Input: part model. Units: mm. Frame: model coordinates. A direction names the side the tool comes from. Round coordinates to 2 decimals unless told otherwise and drop trailing zeros. Write each loop counter-clockwise with the first axis right and the second up, starting at its lowest first coordinate (ties: lowest second). Pieces come first, ordered by that corner, then holes. Notation, with made-up numbers: (-0.75, 16.5) - (56.25, 16.5) arc R23 cw to (56.25, 25.5) - close; hole circle Ø2 at (-19, 16.5). An arc over 180 degrees is marked (long way). Use one line per item in the form item = value.
Autodesk Fusion 360 part; units mm, degrees
sketch "Spacer" plane through (0, 0, 0) normal (0, 1, 0) x (1, 0, 0)
  line L0 (7.0148, 12.15) -> (-7.0148, 12.15)
  line L1 (-7.0148, 12.15) -> (-14.0296, 0)
  line L2 (-14.0296, 0) -> (-7.0148, -12.15)
  line L3 (-7.0148, -12.15) -> (7.0148, -12.15)
  line L4 (7.0148, -12.15) -> (14.0296, 0)
  line L5 (14.0296, 0) -> (7.0148, 12.15)
  line L6 (-12.7883, 22.15) -> (-25.5766, 0)
  line L7 (-25.5766, 0) -> (-12.7883, -22.15)
  line L8 (-12.7883, -22.15) -> (12.7883, -22.15)
  line L9 (12.7883, -22.15) -> (25.5766, 0)
  line L10 (25.5766, 0) -> (12.7883, 22.15)
  line L11 (12.7883, 22.15) -> (-12.7883, 22.15)
  line L12 (-19.1825, 11.075) -> (-10.5222, 6.075) construction
  line L13 (10.5222, 6.075) -> (19.1825, 11.075) construction
  line L14 (10.5222, -6.075) -> (19.1825, -11.075) construction
  line L15 (-10.5222, -6.075) -> (-19.1825, -11.075) construction
  circle A0 centre (-14.8523, 8.575) radius 1.45
  circle A1 centre (14.8523, 8.575) radius 1.45
  circle A2 centre (14.8523, -8.575) radius 1.45
  circle A3 centre (-14.8523, -8.575) radius 1.45
  dimension "d2" = 12.15
  dimension "d3" = 10
  dimension "d5" = 2.9
  dimension "d6" = 2.9
  dimension "d7" = 2.9
  dimension "d8" = 2.9
extrude "Extrude1" add sketch "Spacer" along normal blind 8
sketch "Lock nut hole" plane through (0, 0, 0) normal (0, 1, 0) x (1, 0, 0)
  line L0 (-11.6192, 8.575) -> (-13.2358, 11.375)
  line L1 (-13.2358, 11.375) -> (-16.4689, 11.375)
  line L2 (-16.4689, 11.375) -> (-18.0855, 8.575)
  line L3 (-18.0855, 8.575) -> (-16.4689, 5.775)
  line L4 (-16.4689, 5.775) -> (-13.2358, 5.775)
  line L5 (-13.2358, 5.775) -> (-11.6192, 8.575)
  line L6 (16.4689, 11.375) -> (13.2358, 11.375)
  line L7 (13.2358, 11.375) -> (11.6192, 8.575)
  line L8 (11.6192, 8.575) -> (13.2358, 5.775)
  line L9 (13.2358, 5.775) -> (16.4689, 5.775)
  line L10 (16.4689, 5.775) -> (18.0855, 8.575)
  line L11 (18.0855, 8.575) -> (16.4689, 11.375)
  line L12 (16.4689, -5.775) -> (13.2358, -5.775)
  line L13 (13.2358, -5.775) -> (11.6192, -8.575)
  line L14 (11.6192, -8.575) -> (13.2358, -11.375)
  line L15 (13.2358, -11.375) -> (16.4689, -11.375)
  line L16 (16.4689, -11.375) -> (18.0855, -8.575)
  line L17 (18.0855, -8.575) -> (16.4689, -5.775)
  line L18 (-11.6192, -8.575) -> (-13.2358, -5.775)
  line L19 (-13.2358, -5.775) -> (-16.4689, -5.775)
  line L20 (-16.4689, -5.775) -> (-18.0855, -8.575)
  line L21 (-18.0855, -8.575) -> (-16.4689, -11.375)
  line L22 (-16.4689, -11.375) -> (-13.2358, -11.375)
  line L23 (-13.2358, -11.375) -> (-11.6192, -8.575)
  line L24 (-19.1825, 11.075) -> (-10.5222, 6.075)
  line L25 (10.5222, 6.075) -> (19.1825, 11.075)
  line L26 (-10.5222, -6.075) -> (-19.1825, -11.075)
  line L27 (10.5222, -6.075) -> (19.1825, -11.075)
  point P0 (-14.8523, 8.575)
  point P1 (14.8523, 8.575)
  point P2 (14.8523, -8.575)
  point P3 (-14.8523, -8.575)
  dimension "d11" = 2.8
  dimension "d12" = 2.8
  dimension "d13" = 2.8
  dimension "d14" = 2.8
extrude "Extrude2" [suppressed]
move_body "Move1" [suppressed]
(1) Access query for faces 1 (the face through (11, 8, -10)), 2 (the face through (10.473, 3.944, 6.16)). Directions: +Z, -Z, +X, -X, +Y, -Y. A direction counts if a zero-diameter tool reaches every point of the face in a straight line with its end or side. Return the directions, or none.
Derived:
face_1 = +Z, -Z, +X, -X, +Y
face_2 = +Y, -Y
(2) Draft query along Z for faces 3 (the face through (11, 0, -10)), 4 (the face through (10.57, 3.94, -5.99)), 5 (the face through (0, 4, 22.15)). Return one class per face: released by +Z, released by -Z, zero draft, split by the parting line, or undercut.
Derived:
face_3 = zero draft
face_4 = undercut
face_5 = released by +Z
(3) Material intervals for L1, parallel to Z at x = 0, y = 6.25; L2, parallel to X at y = 7.75, z = -8.5; L3, parallel to Z at x = 13, y = 4.5, sorted ascending.
Derived:
L1 = -22.15 to -12.15, 12.15 to 22.15
L2 = -20.67 to -16.3, -13.4 to -9.12, 9.12 to 13.4, 16.3 to 20.67
L3 = -21.78 to -1.78, 1.78 to 21.78
(4) Cut plane D-D on x = 15. Output: boundary loops of the cut face in (y, z).
Derived:
outline = (0, -18.32) - (8, -18.32) - (8, -10.02) - (0, -10.02) - close; (0, -7.13) - (8, -7.13) - (8, 7.13) - (0, 7.13) - close; (0, 10.02) - (8, 10.02) - (8, 18.32) - (0, 18.32) - close
(5) Cut plane A-A on x = -5. Output: boundary loops of the cut face in (y, z).
Derived:
outline = (0, -22.15) - (8, -22.15) - (8, -12.15) - (0, -12.15) - close; (0, 12.15) - (8, 12.15) - (8, 22.15) - (0, 22.15) - close
(6) First-contact query: pin 1 Ø2.5 at (x, z) = (-14.85, 8.57) entering from +Y; pin 2 Ø4 at (y, z) = (3, -6.5) entering from -X; pin 3 Ø1 at (x, y) = (-20, 1) entering from +Z (3 decimals); pin 4 Ø4 at (x, z) = (7, 11) entering from +Y. Flat tips, straight axial feed; report the tip coordinate or a pass-through.
Derived:
pin_1 = through
pin_2 = -22.98
pin_3 = 10.525
pin_4 = 8
(7) Cut plane B-B on z = 6.5. Output: boundary loops of the cut face in (x, y), then the cut area to 3 significant figures.
Derived:
outline = (-21.82, 0) - (-10.28, 0) - (-10.28, 8) - (-21.82, 8) - close; (10.28, 0) - (21.82, 0) - (21.82, 8) - (10.28, 8) - close
area = 185 mm^2
(8) Cut plane C-C on y = 2. Output: boundary loops of the cut face in (x, z) (3 decimals).
Derived:
outline = (-25.577, 0) - (-12.788, -22.15) - (12.788, -22.15) - (25.577, 0) - (12.788, 22.15) - (-12.788, 22.15) - close; hole circle Ø2.9 at (-14.852, -8.575); hole circle Ø2.9 at (-14.852, 8.575); hole (-14.03, 0) - (-7.015, -12.15) - (7.015, -12.15) - (14.03, 0) - (7.015, 12.15) - (-7.015, 12.15) - close; hole circle Ø2.9 at (14.852, -8.575); hole circle Ø2.9 at (14.852, 8.575)
